The listing builds one solid part. Answer for the finished solid, in the listing's coordinates (mm). Face numbers are marked on the shaded views. A direction names the side the tool comes from. Coordinates: 2 decimals unless noted, no trailing zeros. Order: outer loops, then holes, each group sorted by start corner. A loop starts at its lowest first (then second) coordinate and runs counter-clockwise, first axis right, second up. Notation, with made-up numbers: (-20, 60.25) - (-8, 60.25) arc R24 ccw to (-8, 96.25) - close; hole circle Ø7 at (49, 79.5). An arc over 180 degrees is marked (long way). One line per item, written item: value. Start each with the question number.
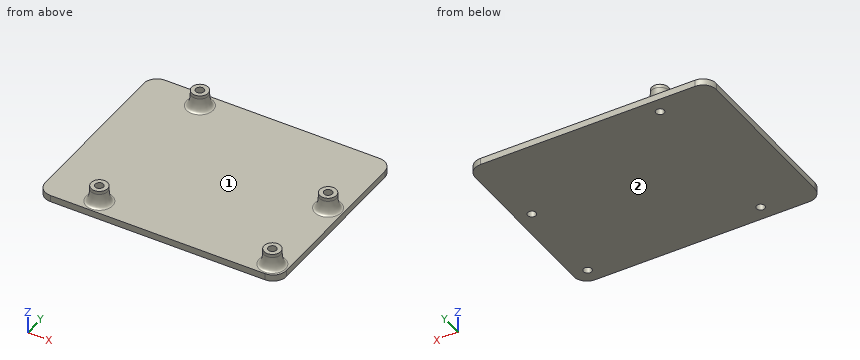
```python
from build123d import *

# Parameters (mm, degrees)
SKETCH1_W           = 68.6
SKETCH1_H           = 53.3
BOSS_EXTRUDE1_DEPTH = 2
SKETCH6_W           = 72.6
SKETCH6_H           = 57.3
BOSS_EXTRUDE3_DEPTH = 2
SKETCH3_R           = 2.5
BOSS_EXTRUDE2_DEPTH = 5
FILLET1_SIZE        = 1.5
FILLET1_SIZE_2      = 4
FILLET2_R           = 4


with BuildPart() as part:
    # Sketch1 → Boss-Extrude1 (new body)
    with BuildSketch(Plane.XY):
        with Locations((16.907139599, -0.839393248)):
            Rectangle(SKETCH1_W, SKETCH1_H)
    extrude(amount=BOSS_EXTRUDE1_DEPTH)

    # Sketch6 → Boss-Extrude3 (add)
    with BuildSketch(Plane.XY.offset(2)):
        with Locations((16.907139599, -0.839393248)):
            Rectangle(SKETCH6_W, SKETCH6_H)
    extrude(amount=-BOSS_EXTRUDE3_DEPTH)

    # Sketch3 → Boss-Extrude2 (add)
    with BuildSketch(Plane.XY.offset(2)):
        with Locations((-2.092860401, 23.210606752)):
            Circle(SKETCH3_R)
    boss_extrude2 = extrude(amount=BOSS_EXTRUDE2_DEPTH)

    # Sketch5 → Tap Drill for M3x0.5 Tap1 (revolve, cut)
    with BuildSketch(Plane(origin=(-2.092860401, 23.210606752, 7), x_dir=(0, -1, 0), z_dir=(1, 0, 0))):
        Polygon((0, 0), (0, 10.751075774), (1.25, 10), (1.25, 0), align=None)
    tap_drill_for_m3x0_5_tap1 = revolve(axis=Axis((-2.092860401, 23.210606752, 13.35), (0, 0, -1)), mode=Mode.SUBTRACT)

    # Sketch-Pattern1: Boss-Extrude2, Tap Drill for M3x0.5 Tap1 at 3 more places
    with Locations((50.8, -48.2, 0), (-1.3, -48.2, 0), (50.8, -20.3, 0)):
        add(boss_extrude2)
        add(tap_drill_for_m3x0_5_tap1, mode=Mode.SUBTRACT)

    # Fillet1
    # an asymmetric fillet: 4, 1.5 mm, written as the material it adds along each edge
    with BuildSketch(Plane(origin=(-2.092860401, 23.210606752, 2), x_dir=(1, 0, 0), z_dir=(0, -1, 0))) as fillet1_piece_1:
        with BuildLine():
            Bezier((2.5 + FILLET1_SIZE, 0), (2.5, 0), (2.5, FILLET1_SIZE_2), weights=[1, 0.707106781, 1])
            Line((2.5, FILLET1_SIZE_2), (2.5, 0))
            Line((2.5, 0), (2.5 + FILLET1_SIZE, 0))
        make_face()
    revolve(axis=Axis((-2.092860401, 23.210606752, 2), (0, 0, 1)))
    with BuildSketch(Plane(origin=(48.707139599, -24.989393248, 2), x_dir=(1, 0, 0), z_dir=(0, -1, 0))) as fillet1_piece_2:
        with BuildLine():
            Bezier((2.5 + FILLET1_SIZE, 0), (2.5, 0), (2.5, FILLET1_SIZE_2), weights=[1, 0.707106781, 1])
            Line((2.5, FILLET1_SIZE_2), (2.5, 0))
            Line((2.5, 0), (2.5 + FILLET1_SIZE, 0))
        make_face()
    revolve(axis=Axis((48.707139599, -24.989393248, 2), (0, 0, 1)))
    with BuildSketch(Plane(origin=(-3.392860401, -24.989393248, 2), x_dir=(1, 0, 0), z_dir=(0, -1, 0))) as fillet1_piece_3:
        with BuildLine():
            Bezier((2.5 + FILLET1_SIZE, 0), (2.5, 0), (2.5, FILLET1_SIZE_2), weights=[1, 0.707106781, 1])
            Line((2.5, FILLET1_SIZE_2), (2.5, 0))
            Line((2.5, 0), (2.5 + FILLET1_SIZE, 0))
        make_face()
    revolve(axis=Axis((-3.392860401, -24.989393248, 2), (0, 0, 1)))
    with BuildSketch(Plane(origin=(48.707139599, 2.910606752, 2), x_dir=(1, 0, 0), z_dir=(0, -1, 0))) as fillet1_piece_4:
        with BuildLine():
            Bezier((2.5 + FILLET1_SIZE, 0), (2.5, 0), (2.5, FILLET1_SIZE_2), weights=[1, 0.707106781, 1])
            Line((2.5, FILLET1_SIZE_2), (2.5, 0))
            Line((2.5, 0), (2.5 + FILLET1_SIZE, 0))
        make_face()
    revolve(axis=Axis((48.707139599, 2.910606752, 2), (0, 0, 1)))

    # Fillet2
    fillet2_edges = [part.edges().sort_by_distance(p)[0] for p in [
        (-19.392860401, 27.810606752, 1),
        (53.207139599, 27.810606752, 1),
        (53.207139599, -29.489393248, 1),
        (-19.392860401, -29.489393248, 1),
    ]]
    fillet(fillet2_edges, radius=FILLET2_R)


solid = part.part
```
(1) The part is cut by section B-B on x = 4. Determine the outline of the cut face in (y, z), plus the area to 3 significant figures.
(2) For the marked faces 1 and 2, determine the directions among +Z, -Z, +X, -X, +Y, -Y from which every point of the face is accessible in a straight line to the end or side of a thin tool.
(3) Flat-ended cylindrical pins translate along their axes: pin 1 Ø1 at (y, z) = (-20.5, 5.5) entering from -X; pin 2 Ø3 at (x, y) = (-3.39, -24.99) entering from +Z; pin 3 Ø1 at (x, y) = (17, 0.5) entering from +Z. Find the tip coordinate at first contact, or state that the pin passes through.
(4) The part is cut by section C-C on y = 14. Determine the outline of the cut face in (x, z).
(5) The part is cut by section A-A on z = 5. Count the separate pieces of the cut face and the enclosed holes in it, plus the area to 3 significant figures.
(6) Consider probe 1 along Z at (x, y) = (15, -9); probe 2 along X at (y, z) = (-23.5, 5.25); probe 3 along Y at (x, z) = (-1.5, 1.5). Determine where each line is inside the solid, lowest interval first.
Completed:
1. outline: (-29.49, 0) - (27.81, 0) - (27.81, 2) - (-29.49, 2) - close
1. area: 115 mm2
2. face 1: +Z
2. face 2: -Z, +X, -X, +Y, -Y
3. pin 1: passes through
3. pin 2: stops at z = 7
3. pin 3: stops at z = 2
4. outline: (-19.39, 0) - (53.21, 0) - (53.21, 2) - (-19.39, 2) - close
5. separate pieces: 4
5. enclosed holes: 4
5. area: 61.9 mm2
6. probe 1: z = 0 to 2
6. probe 2: x = -5.43 to -1.35, 46.67 to 50.75
6. probe 3: y = -29.49 to 22.11, 24.31 to 27.81
